```python
from build123d import *

# Parameters (mm, degrees)
SKETCH1_R           = 1.75
BOSS_EXTRUDE1_DEPTH = 10
SKETCH2_R           = 1.5
CUT_EXTRUDE1_DEPTH  = 15
SKETCH3_R           = 4.25
SKETCH3_R_2         = 3.25
CUT_EXTRUDE2_DEPTH  = 354.694783677


with BuildPart() as part:
    # Sketch1 → Boss-Extrude1 (new body)
    with BuildSketch(Plane(origin=(0, 0, 0), x_dir=(0, 0, -1), z_dir=(1, 0, 0))):
        Polygon((50, 0), (125, 0), (125, -10), (175, -10), (175, 0), (225, 0), (250, 25), (250, 200), (200, 250), (0, 250), (0, 125), (-10, 125), (-10, 75), (0, 75), (0, 50), align=None)
        with Locations((-5, 113)):
            Circle(SKETCH1_R, mode=Mode.SUBTRACT)
        with Locations((-5, 87)):
            Circle(SKETCH1_R, mode=Mode.SUBTRACT)
        with Locations((137, -5)):
            Circle(SKETCH1_R, mode=Mode.SUBTRACT)
        with Locations((163, -5)):
            Circle(SKETCH1_R, mode=Mode.SUBTRACT)
    extrude(amount=BOSS_EXTRUDE1_DEPTH)

    # Sketch2 → Cut-Extrude1 (cut)
    with BuildSketch(Plane(origin=(0, 225, -225), x_dir=(1, 0, 0), z_dir=(0, 0.7071067811865477, -0.7071067811865475))):
        with Locations(Location((5, 4.644660941, 0), (0, 0, 270))):
            Circle(SKETCH2_R)
        with Locations(Location((5, -25.355339059, 0), (0, 0, 270))):
            Circle(SKETCH2_R)
    extrude(amount=-CUT_EXTRUDE1_DEPTH, mode=Mode.SUBTRACT)

    # Sketch3 → Cut-Extrude2 (cut, through all)
    with BuildSketch(Plane(origin=(10, 0, 0), x_dir=(0, 0, -1), z_dir=(1, 0, 0))):
        with Locations((230, 50)):
            Circle(SKETCH3_R)
        with Locations((200, 20)):
            Circle(SKETCH3_R_2)
    extrude(amount=-CUT_EXTRUDE2_DEPTH, mode=Mode.SUBTRACT)


solid = part.part
```
Work out the finished part from the listing and answer in its coordinate system (mm). A direction names the side the tool comes from. Give positions to 0.01 mm unless a question says otherwise; leave off trailing zeros. Loops run counter-clockwise (first coordinate to the right, second up) from the corner with the lowest first, then second, coordinate; pieces in that order, holes last. Notation, with made-up numbers: M 74.25,30 L 97.25,30 A4 ccw 97.25,35 Z; hole C 4.5,19.25 d11. An arc over 180 degrees is marked long. One line per item, written item: value. Start each with the question number.
1. Which of the six approach directions +Z, -Z, +X, -X, +Y, -Y give full straight-line access (tool end or side, diameter ignored) to faces 1 (the face through (5, 75, 5)), 2 (the face through (10, 122, -118)), 3 (the face through (5, 111, -250)), 4 (the face through (5, 125, 5)), 5 (the face through (5, -5, -175))?
2. Find section A-A (y = 20). Give the vertices of the cut face in (x, z), and give its area (4 significant figures).
3. Each of these flat-tipped pins is pushed along its axis until it touches: P1, Ø10.5, axis at y = 20, z = -200, coming from the +X side; P2, Ø3, axis at x = 7, z = 3.5, coming from the -Y side; P3, Ø5, axis at x = 4, y = -6.5, coming from the +Z side; P4, Ø5, axis at x = 7, z = -196, coming from the -Y side. Where does it stop, or does it pass through?
4. Find the intervals of material crossed by probe 1 along Z at (x, y) = (6.75, 87); probe 2 along Y at (x, z) = (5.5, -137); probe 3 along Y at (x, z) = (5.75, -60), in increasing order.
5. Find section C-C (y = 182.5). Give the vertices of the cut face in (x, z), and give its area (3 significant figures).
6. Determine the mould class of faces 6 (the face through (5, 250, -101)), 7 (the face through (5, 188, 0)), 8 (the face through (4.425, 217.466, -222.075)) for opening direction Z: released by +Z, released by -Z, zero draft, split by the parting line, or undercut.
7. Find section B-B (x = 1.75). Give the vertices of the cut face in (y, z), and give its area (3 significant figures).
Reported:
1. face 1: +Z, +X, -X, -Y
1. face 2: +Z, -Z, +X, +Y, -Y
1. face 3: -Z, +X, -X, +Y, -Y
1. face 4: +Z, +X, -X, +Y
1. face 5: -Z, +X, -X, -Y
2. outline: M 0,-245 L 10,-245 L 10,-203.25 L 0,-203.25 Z; M 0,-196.75 L 10,-196.75 L 10,-30 L 0,-30 Z
2. area: 2,085 mm²
3. P1: stops at x = 10
3. P2: stops at y = 75
3. P3: stops at z = -125
3. P4: stops at y = 0
4. probe 1: z = -250 to 3.25, 6.75 to 10
4. probe 2: y = -10 to -6.75, -3.25 to 250
4. probe 3: y = 0 to 250
5. outline: M 0,-250 L 10,-250 L 10,0 L 0,0 Z
5. area: 2,500 mm²
6. face 6: zero draft
6. face 7: released by +Z
6. face 8: undercut
7. outline: M -10,-175 L 0,-175 L 0,-225 L 25,-250 L 200,-250 L 250,-200 L 250,0 L 125,0 L 125,10 L 75,10 L 75,0 L 50,0 L 0,-50 L 0,-125 L -10,-125 Z; hole C -5,-163 d3.5; hole C -5,-137 d3.5; hole C 20,-200 d6.5; hole C 50,-230 d8.5; hole C 87,5 d3.5; hole C 113,5 d3.5
7. area: 60,600 mm²
